Autodesk Inventor part; units mm, degrees
ref_plane "YZ Plane" through (0, 0, 0) normal (1, 0, 0) x (0, 1, 0)
ref_plane "XZ Plane" through (0, 0, 0) normal (0, 1, 0) x (-1, 0, 0)
ref_plane "XY Plane" through (0, 0, 0) normal (0, 0, 1) x (1, 0, 0)
sketch "Sketch1" plane through (0, 0, 0) normal (0, 1, 0) x (-1, 0, 0)
  circle A0 centre (0, 0) radius 4
  circle A1 centre (0, 0) radius 7
  dimension "d0" = 8
  dimension "d1" = 3
extrude "Extrusion1" add sketch "Sketch1" along normal blind 20 contours A0 | A1
sketch "Sketch2" plane through (0, 20, 0) normal (0, 1, 0) x (1, 0, 0)
  circle A0 centre (0, 0) radius 3.175
  dimension "d4" = 6.35
extrude "Extrusion2" cut sketch "Sketch2" against normal blind 10
extrude "Extrusion3" cut sketch "Sketch1" along normal blind 10 contours A0
properties part number "mixer_coupler"
Could you check a few things on this model? Use its own coordinates, in mm. A direction names the side the tool comes from. Round coordinates to 2 decimals unless told otherwise and drop trailing zeros. Loops run counter-clockwise (first coordinate to the right, second up) from the corner with the lowest first, then second, coordinate; pieces in that order, holes last. Notation, with made-up numbers: (45, -25) - (98, -25) arc R25 ccw to (98, 4) - close; hole circle Ø7 at (-36.75, 0). An arc over 180 degrees is marked (long way). Answer in a Markdown table with one row per item. Add a question column.
(1) If we section it at D-D (y = 17): Please give me the cut outline in (x, z) (3 decimals), plus the area to 3 significant figures.
(2) I need wall thicknesses on line 1 along Z through (x, y) = (0, 13.5) (3 decimals); line 2 along Z through (x, y) = (0, 5); line 3 along Y through (x, z) = (-2, -2.5). Which ranges of each line are inside material? Lowest first, please.
(3) If we section it at C-C (y = 8.5): Please give me the cut outline in (x, z).
(4) If we section it at B-B (x = 0): Please give me the cut outline in (y, z) (3 decimals), plus the area to 4 significant figures.
(5) If we section it at A-A (z = 0): Please give me the cut outline in (x, y) (3 decimals), plus the area to 4 significant figures.
(6) If we mould it in two halves opening along Z, with no side actions, what happens to faces 3 (the face through (-6.466, 9.86, 2.681)), 4 (the face through (-1.5, 20, -3)), 5 (the face through (-0.69, 15.07, 3.1))? For each: pulls with the +Z half, pulls with the -Z half, needs draft (parallel to the pull), parting line crosses it, or undercut.
(7) I'm going to push flat-ended pins straight in: pin 1 (1 mm diameter, centred on x = 1, z = 4, fed in from -Y); pin 2 (5 mm diameter, centred on x = 0, z = 0, fed in from -Y); pin 3 (6.5 mm diameter, centred on x = -0.5, z = 0, fed in from -Y); pin 4 (6 mm diameter, centred on x = -5, y = 7.5, fed in from -Z). Where does each tip first touch, or does it pass through?
(8) For faces 1 (the face through (-3, 0, -3)), 2 (the face through (0.867, 4.93, 3.905)), which set-ups out of +Z, -Z, +X, -X, +Y, -Y let a thin tool reach every point of the face, with its end or its side?
Model answer:
| question | item | result |
|---|---|---|
| 1 | outline | circle Ø14 at (0, 0); hole circle Ø6.35 at (0, 0) |
| 1 | area | 122 mm² |
| 2 | line 1 | z = -7 to -3.175, 3.175 to 7 |
| 2 | line 2 | z = -7 to -4, 4 to 7 |
| 2 | line 3 | y = 10 to 20 |
| 3 | outline | circle Ø14 at (0, 0); hole circle Ø8 at (0, 0) |
| 4 | outline | (0, -7) - (20, -7) - (20, -3.175) - (10, -3.175) - (10, -4) - (0, -4) - close; (0, 4) - (10, 4) - (10, 3.175) - (20, 3.175) - (20, 7) - (0, 7) - close |
| 4 | area | 136.5 mm² |
| 5 | outline | (-7, 0) - (-4, 0) - (-4, 10) - (-3.175, 10) - (-3.175, 20) - (-7, 20) - close; (3.175, 10) - (4, 10) - (4, 0) - (7, 0) - (7, 20) - (3.175, 20) - close |
| 5 | area | 136.5 mm² |
| 6 | face 3 | parting line crosses it |
| 6 | face 4 | needs draft |
| 6 | face 5 | undercut |
| 7 | pin 1 | stops at y = 0 |
| 7 | pin 2 | passes through |
| 7 | pin 3 | stops at y = 10 |
| 7 | pin 4 | stops at z = -6.71 |
| 8 | face 1 | +Z, -Z, +X, -X, -Y |
| 8 | face 2 | -Y |
